Job drawing, mm, ordinate dimensions from the low corner. One solid piece. A direction names the side the tool comes from. Give positions to 0.01 mm unless a question says otherwise; leave off trailing zeros. Loops run counter-clockwise (first coordinate to the right, second up) from the corner with the lowest first, then second, coordinate; pieces in that order, holes last. Notation, with made-up numbers: M -4.5,41.5 L 12.5,41.5 A24 cw 12.5,55.5 Z; hole C -39,10 d8. An arc over 180 degrees is marked long. One line per question, with ' | ' between items.
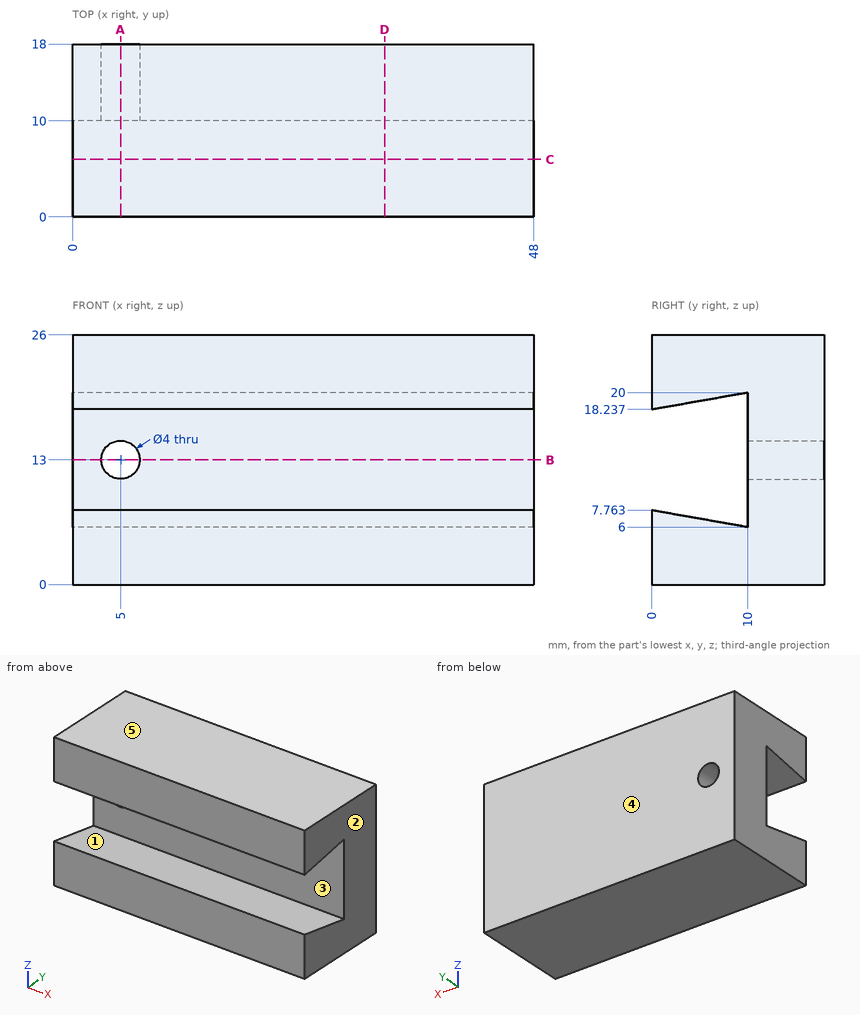
Item 1: Drill centre lines: line 1 along X through (y, z) = (15.25, 13); line 2 along Z through (x, y) = (5, 15.75); line 3 along Y through (x, z) = (16.5, 13). Where is each one in solid material? Low to high. Write a range as [from, to].
Conclusion:
line 1: [0, 3], [7, 48] | line 2: [0, 11], [15, 26] | line 3: [10, 18]
Item 2: Drop a flat-ended pin along its axis: P1, Ø10, axis at y = 9, z = 14.5, coming from the +X side. Give the stop position or say it passes through.
Conclusion:
P1: x = 48
Item 3: Saw through at B-B on z = 13. Give the cut face in (x, y), and give its area (3 significant figures).
Conclusion:
outline: M 0,10 L 3,10 L 3,18 L 0,18 Z; M 7,10 L 48,10 L 48,18 L 7,18 Z | area: 352 mm²
Item 4: Saw through at A-A on x = 5. Give the cut face in (y, z).
Conclusion:
outline: M 0,0 L 18,0 L 18,11 L 10,11 L 10,6 L 0,7.76 Z; M 0,18.24 L 10,20 L 10,15 L 18,15 L 18,26 L 0,26 Z
Item 5: Mould opens along Z. For the marked faces 3, 4 and 5 say: pulls with the +Z half, pulls with the -Z half, needs draft (parallel to the pull), parting line crosses it, or undercut.
Conclusion:
face 3: undercut | face 4: needs draft | face 5: pulls with the +Z half
Item 6: 3-axis set-ups, long thin cutter, end or side, ignore diameter. For the marked faces 1 and 2: which of +Z, -Z, +X, -X, +Y, -Y reach the whole face in a straight line?
Conclusion:
face 1: +X, -X | face 2: +Z, -Z, +X, +Y, -Y
Item 7: Saw through at C-C on y = 6. Give the cut face in (x, z) (1 decimal).
Conclusion:
outline: M 0,0 L 48,0 L 48,6.7 L 0,6.7 Z; M 0,19.3 L 48,19.3 L 48,26 L 0,26 Z
Item 8: Saw through at D-D on x = 32.5. Give the cut face in (y, z).
Conclusion:
outline: M 0,0 L 18,0 L 18,26 L 0,26 L 0,18.24 L 10,20 L 10,6 L 0,7.76 Z
